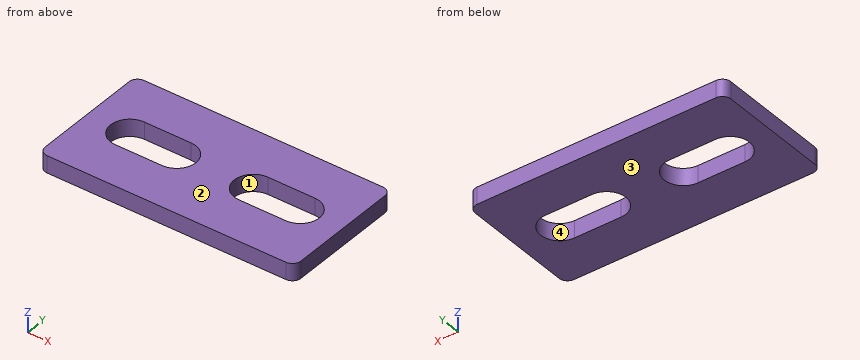
Autodesk Inventor part; units mm, degrees
ref_plane "YZ Plane" through (0, 0, 0) normal (1, 0, 0) x (0, 1, 0)
ref_plane "XZ Plane" through (0, 0, 0) normal (0, 1, 0) x (-1, 0, 0)
ref_plane "XY Plane" through (0, 0, 0) normal (0, 0, 1) x (1, 0, 0)
sketch "Náčrt1" plane through (0, 0, 0) normal (0, 0, 1) x (1, 0, 0)
  line L0 (-42, 0) -> (42, 0)
  line L1 (0, -21) -> (0, 21)
  line L2 (30, -15) -> (-30, -15)
  line L3 (-30, -15) -> (-30, 15)
  line L4 (-30, 15) -> (30, 15)
  line L5 (30, 15) -> (30, -15)
  point P0 (0, 0)
  dimension "d0" = 60
  dimension "d1" = 30
extrude "Vysunutí1" add sketch "Náčrt1" along normal blind 4
sketch "Náčrt2" plane through (0, 0, 4) normal (0, 0, 1) x (1, 0, 0)
  line L0 (30, 15) -> (-30, 15)
  line L1 (-30, 15) -> (-30, -15)
  line L2 (-30, -15) -> (30, -15)
  line L3 (30, -15) -> (30, 15)
  line L4 (-42, 0) -> (42, 0)
  line L5 (0, -21) -> (0, 21)
  line L6 (-20, 0) -> (-9, 0) construction
  line L7 (-20, -4.5) -> (-9, -4.5)
  line L8 (-9, 4.5) -> (-20, 4.5)
  arc A0 (-20, 4.5) -> (-20, -4.5) centre (-20, 0) ccw
  arc A1 (-9, -4.5) -> (-9, 4.5) centre (-9, 0) ccw
  point P0 (0, 0)
  point P1 (-14.5, 0)
  dimension "d4" = 9
  dimension "d5" = 11
  dimension "d6" = 10
extrude "Vysunutí2" cut sketch "Náčrt2" against normal through all contours A1 L7 A0 L4 | L4 A0 L8 A1
mirror "Zrcadlit1" about plane through (0, 0, 0) normal (1, 0, 0) of "Vysunutí2"
fillet "Zaoblení1" radius 2 4 edges at (-30, 15, 2) (30, 15, 2) (30, -15, 2) (-30, -15, 2)
properties part number "connector_30x30"
Model file for the job. Use its own axes, mm. Face numbers are marked on the shaded views. A direction names the side the tool comes from. Give positions to 0.01 mm unless a question says otherwise; leave off trailing zeros. Order: outer loops, then holes, each group sorted by start corner. A loop starts at its lowest first (then second) coordinate and runs counter-clockwise, first axis right, second up. Notation, with made-up numbers: M 85,32 L 93,32 A35 ccw 93,69 Z; hole C 16.25,15 d1. An arc over 180 degrees is marked long. Put each result on its own line as item: value. Start each with the question number.
(1) Band-saw the part on B-B on y = 0. Give the cut face in (x, z).
(2) Band-saw the part on C-C on x = -16. Give the cut face in (y, z).
(3) Pin check, flat tip, straight feed: pin 1 Ø4 at (x, y) = (-6, -4) entering from -Z. Stop position of the tip, or through.
(4) Drill centre lines: L1, parallel to Y at x = -9, z = 0.85; L2, parallel to X at y = 1, z = 0.75; L3, parallel to Y at x = 6, z = 2.4. Where is each one in solid material? Low to high. Write a range as [from, to].
(5) Pull direction Y, two halves, no side cores. Call the marked faces 1 and 2: released by +Y, released by -Y, zero draft, split by the parting line, or undercut.
(6) Tool access for the marked faces 3 and 4: list every direction of +Z, -Z, +X, -X, +Y, -Y with a clear straight run to the whole face (end or side of a thin tool).
(7) Band-saw the part on A-A on x = -7.5. Give the cut face in (y, z), then the cut area to 3 significant figures.
Results below:
1. outline: M -30,0 L -24.5,0 L -24.5,4 L -30,4 Z; M -4.5,0 L 4.5,0 L 4.5,4 L -4.5,4 Z; M 24.5,0 L 30,0 L 30,4 L 24.5,4 Z
2. outline: M -15,0 L -4.5,0 L -4.5,4 L -15,4 Z; M 4.5,0 L 15,0 L 15,4 L 4.5,4 Z
3. pin 1: stops at z = 0
4. L1: y = [-15, -4.5], [4.5, 15]
4. L2: x = [-30, -24.39], [-4.61, 4.61], [24.39, 30]
4. L3: y = [-15, -3.35], [3.35, 15]
5. face 1: undercut
5. face 2: zero draft
6. face 3: -Z, +X, -X, +Y, -Y
6. face 4: +Z, -Z
7. outline: M -15,0 L -4.24,0 L -4.24,4 L -15,4 Z; M 4.24,0 L 15,0 L 15,4 L 4.24,4 Z
7. area: 86.1 mm2
